Geometry check sheet. Reference: the model listing, model coordinates, mm. A direction names the side the tool comes from. Coordinates: 2 decimals unless noted, no trailing zeros. Loops run counter-clockwise (first coordinate to the right, second up) from the corner with the lowest first, then second, coordinate; pieces in that order, holes last. Notation, with made-up numbers: (4, 37) -> (30, 37) arc R15 ccw to (30, 57) -> close; hole circle Ø10 at (42, 30). An arc over 180 degrees is marked (long way). Answer as a JSON object with one key per item and string values.
from build123d import *

# Parameters (mm, degrees)
SKETCH_1_W          = 28
SKETCH_1_H          = 12
EXTRUDE_1_DEPTH     = 31
FILLET_1_R          = 6
SKETCH_2_R          = 3
EXTRUDE_2_DEPTH     = 14
SKETCH_3_W          = 11
SKETCH_3_H          = 2.5
EXTRUDE_3_DEPTH     = 4
SKETCH_4_W          = 11
SKETCH_4_H          = 1
EXTRUDE_4_DEPTH     = 10
EXTRUDE_5_DEPTH     = 11
SKETCH_7_R          = 4.985468992
CUT_EXTRUDE_1_DEPTH = 1


with BuildPart() as part:
    # ｽｹｯﾁ1 → ﾎﾞｽ - 押し出し1 (new body)
    with BuildSketch(Plane.XY):
        with Locations((14, 6)):
            Rectangle(SKETCH_1_W, SKETCH_1_H)
    extrude(amount=EXTRUDE_1_DEPTH)

    # ﾌｨﾚｯﾄ1
    fillet_1_edges = [part.edges().sort_by_distance(p)[0] for p in [
        (28, 0, 15.5),
        (28, 12, 15.5),
        (0, 0, 15.5),
        (0, 12, 15.5),
    ]]
    fillet(fillet_1_edges, radius=FILLET_1_R - 0.0001)  # a hair under: the kernel refuses the full size

    # ｽｹｯﾁ2 → ﾎﾞｽ - 押し出し2 (add)
    with BuildSketch(Plane.XY.offset(31)):
        with Locations(Location((14, 6, 0), (0, 0, 180))):
            Circle(SKETCH_2_R)
        with Locations(Location((6.799424136, 6, 0), (0, 0, 180))):
            Circle(SKETCH_2_R)
        with Locations(Location((21.200575864, 6, 0), (0, 0, 180))):
            Circle(SKETCH_2_R)
    extrude(amount=EXTRUDE_2_DEPTH)

    # ｽｹｯﾁ3 → ﾎﾞｽ - 押し出し3 (add)
    with BuildSketch(Plane(origin=(0, 12, 0), x_dir=(1, 0, 0), z_dir=(0, 1, 0))):
        with Locations((14.202566522, -21.75)):
            Rectangle(SKETCH_3_W, SKETCH_3_H)
    extrude(amount=EXTRUDE_3_DEPTH)

    # ｽｹｯﾁ4 → ﾎﾞｽ - 押し出し4 (add)
    with BuildSketch(Plane.XY.offset(23)):
        with Locations((14.202566522, 15.5)):
            Rectangle(SKETCH_4_W, SKETCH_4_H)
    extrude(amount=EXTRUDE_4_DEPTH)

    # ｽｹｯﾁ6 → ﾎﾞｽ - 押し出し5 (add)
    with BuildSketch(Plane(origin=(19.702566522, 0, 0), x_dir=(0, 0, -1), z_dir=(1, 0, 0))):
        with BuildLine():
            Line((-32.878667376, 17.912838666), (-34.912838666, 17.912838666))
            ThreePointArc((-34.912838666, 17.912838666), (-33.572911973, 17.339926693), (-33, 16))
            Line((-33, 16), (-30.566032893, 16))
            Line((-30.566032893, 16), (-32.247451697, 17.654373362))
            ThreePointArc((-32.247451697, 17.654373362), (-32.537625756, 17.845719578), (-32.878667376, 17.912838666))
        make_face()
    extrude(amount=-EXTRUDE_5_DEPTH)

    # ｽｹｯﾁ7 → ｶｯﾄ - 押し出し1 (cut)
    with BuildSketch(Plane(origin=(0, 0, 0), x_dir=(-1, 0, 0), z_dir=(0, 0, -1))):
        with Locations((-14, 6.447278685)):
            Circle(SKETCH_7_R)
    extrude(amount=-CUT_EXTRUDE_1_DEPTH, mode=Mode.SUBTRACT)


solid = part.part
1. Section check C-C, the plane z = 42. Record the boundary of the cut face in (x, y).
Evaluation:
{"outline": "circle Ø6 at (6.8, 6); circle Ø6 at (14, 6); circle Ø6 at (21.2, 6)"}
2. Section check A-A, the plane x = 14. Record the boundary of the cut face in (y, z), then the cut area to 3 significant figures.
Evaluation:
{"outline": "(0, 0) -> (1.46, 0) -> (1.46, 1) -> (11.43, 1) -> (11.43, 0) -> (12, 0) -> (12, 20.5) -> (16, 20.5) -> (16, 30.57) -> (17.65, 32.25) arc R0.9 ccw to (17.91, 32.88) -> (17.91, 34.91) arc R1.96 cw to (16, 33) -> (15, 33) -> (15, 23) -> (12, 23) -> (12, 31) -> (9, 31) -> (9, 45) -> (3, 45) -> (3, 31) -> (0, 31) -> close", "area": "470 mm^2"}
3. Section check D-D, the plane y = 9.5. Record the boundary of the cut face in (x, z).
Evaluation:
{"outline": "(1.13, 0) -> (10.06, 0) -> (10.06, 1) -> (17.94, 1) -> (17.94, 0) -> (26.87, 0) -> (26.87, 31) -> (1.13, 31) -> close"}
4. Tool access check on faces 1 (the face through (14.1, 15.5, 33)), 2 (the face through (14, 7, 1)), 3 (the face through (19.703, 15.2, 26.1)), 4 (the face through (14, 16, 25)). Record the directions out of +Z, -Z, +X, -X, +Y, -Y that give a thin tool (end or side, any length) a straight path to the whole face; none if there is none.
Evaluation:
{"face 1": "+Z, +X, -X", "face 2": "-Z", "face 3": "+Z, -Z, +X, +Y", "face 4": "-Z, +X, -X, +Y"}
5. Mould release check, pull along X, two halves, no side actions. Record for faces 5 (the face through (24.2, 5.9, 37.9)), 6 (the face through (9.245, 7.945, 0.493)), 7 (the face through (14, 13, 23)), 8 (the face through (26.289, 10.196, 15.717)): released by +X, released by -X, zero draft, split by the parting line, or undercut.
Evaluation:
{"face 5": "undercut", "face 6": "undercut", "face 7": "zero draft", "face 8": "released by +X"}
6. Depth check by flat-ended pin: P1, Ø1.1, axis at x = 13.5, y = 15.5, coming from the +Z side; P2, Ø8, axis at x = 12, y = 6.5, coming from the -Z side; P3, Ø1.8, axis at y = 13.5, z = 24.5, coming from the +X side; P4, Ø13, axis at x = 16, z = 8, coming from the +Y side. Enter the tip coordinate at first touch or a pass-through.
Evaluation:
{"P1": "stops at z = 33", "P2": "stops at z = 0", "P3": "passes through", "P4": "stops at y = 12"}
7. Thickness scan on probe 1 along Y at (x, z) = (14, 0.65); probe 2 along Y at (x, z) = (18, 29); probe 3 along X at (y, z) = (14.5, 22.5). Record the ranges inside material, lowest first. Write a range as from..to.
Evaluation:
{"probe 1": "y = 0..1.46, 11.43..12", "probe 2": "y = 0..12, 15..16", "probe 3": "x = 8.7..19.7"}
